The listing builds one solid part. Answer for the finished solid, in the listing's coordinates (mm). Coordinates: 2 decimals unless noted, no trailing zeros. Loops run counter-clockwise (first coordinate to the right, second up) from the corner with the lowest first, then second, coordinate; pieces in that order, holes last. Notation, with made-up numbers: (1.25, -14) - (35.25, -14) arc R35 ccw to (35.25, 23) - close; hole circle Ø4 at (-21.5, 84.5). An arc over 180 degrees is marked (long way). Write each question's results on one line, items separated by ' | '. Start each with the question number.
(1) Consider line 1 (Z direction, x = 31.5, y = 1.15); line 2 (Y direction, x = -5.5, z = 97). Determine where each line is inside the solid, lowest interval first. Write a range as from..to.
(2) Find section B-B on y = 0.8. Determine the outline of the cut face in (x, z).
(3) Find section A-A on x = 57. Determine the outline of the cut face in (y, z).
(4) Given pin 1 Ø1.5 at (x, y) = (-27, 1) entering from -Z; pin 2 Ø0.6 at (x, y) = (-23.5, 1) entering from +Z; pin 3 Ø3 at (x, z) = (-31.5, -99.5) entering from -Y, each flat-ended and moving along its own axis, determine where each tip first touches the part or whether it passes through.
from build123d import *

# Parameters (mm, degrees)
SKETCH2_W               = 140
SKETCH2_H               = 420
BOSS_EXTRUDE1_DEPTH     = 4
BOSS_EXTRUDE2_DEPTH     = 25
SKETCH4_W               = 10.25
SKETCH4_H               = 80.25
CUT_EXTRUDE1_DEPTH      = 25.4
SKETCH7_W               = 130
SKETCH7_H               = 10
CUT_EXTRUDE2_DEPTH      = 2.45
SKETCH9_W               = 140
SKETCH9_H               = 115
SKETCH9_W_2             = 10.25
SKETCH9_H_2             = 80.25
CUT_EXTRUDE3_DEPTH      = 1
CUT_EXTRUDE3_DEPTH_BACK = 30
SKETCH10_W              = 140
SKETCH10_H              = 10
BOSS_EXTRUDE3_DEPTH     = 2


with BuildPart() as part:
    # Sketch2 → Boss-Extrude1 (new body)
    with BuildSketch(Plane(origin=(0, 0, 0), x_dir=(1, 0, 0), z_dir=(0, 1, 0))):
        Rectangle(SKETCH2_W, SKETCH2_H)
    extrude(amount=BOSS_EXTRUDE1_DEPTH)

    # Sketch3 → Boss-Extrude2 (add)
    with BuildSketch(Plane(origin=(0, 4, 0), x_dir=(1, 0, 0), z_dir=(0, 1, 0))):
        with BuildLine():
            Line((-37.5, -165), (-37.5, -145))
            Line((-37.5, -145), (-43.5, -145))
            Line((-43.5, -145), (-43.5, -165))
            ThreePointArc((-43.5, -165), (0, -208.5), (43.5, -165))
            Line((43.5, -165), (43.5, -145))
            Line((43.5, -145), (37.5, -145))
            Line((37.5, -145), (37.5, -165))
            ThreePointArc((37.5, -165), (0, -202.5), (-37.5, -165))
        make_face()
    extrude(amount=BOSS_EXTRUDE2_DEPTH)

    # Sketch4 → Cut-Extrude1 (cut)
    with BuildSketch(Plane(origin=(0, 4, 0), x_dir=(1, 0, 0), z_dir=(0, 1, 0))):
        with Locations((-59.875, 139.875)):
            Rectangle(SKETCH4_W, SKETCH4_H)
        with Locations((59.875, 139.875)):
            Rectangle(SKETCH4_W, SKETCH4_H)
    extrude(amount=-CUT_EXTRUDE1_DEPTH, mode=Mode.SUBTRACT)

    # Sketch7 → Cut-Extrude2 (cut)
    with BuildSketch(Plane(origin=(0, 4, 0), x_dir=(1, 0, 0), z_dir=(0, 1, 0))):
        with Locations((0, 200)):
            Rectangle(SKETCH7_W, SKETCH7_H)
    extrude(amount=-CUT_EXTRUDE2_DEPTH, mode=Mode.SUBTRACT)

    # Sketch9 → Cut-Extrude3 (cut, two sides)
    with BuildSketch(Plane.XZ) as cut_extrude3_sk:
        with Locations((0, 152.5)):
            Rectangle(SKETCH9_W, SKETCH9_H)
        with Locations((0, -152.5)):
            Rectangle(SKETCH9_W, SKETCH9_H)
        with Locations((-59.875, -139.875)):
            Rectangle(SKETCH9_W_2, SKETCH9_H_2, mode=Mode.SUBTRACT)
        with Locations((59.875, -139.875)):
            Rectangle(SKETCH9_W_2, SKETCH9_H_2, mode=Mode.SUBTRACT)
    extrude(amount=CUT_EXTRUDE3_DEPTH, mode=Mode.SUBTRACT)
    extrude(cut_extrude3_sk.sketch, amount=-CUT_EXTRUDE3_DEPTH_BACK, mode=Mode.SUBTRACT)

    # Sketch10 → Boss-Extrude3 (add)
    with BuildSketch(Plane(origin=(0, 4, 0), x_dir=(1, 0, 0), z_dir=(0, 1, 0))):
        with Locations((0, 100)):
            Rectangle(SKETCH10_W, SKETCH10_H)
        with Locations((0, -100)):
            Rectangle(SKETCH10_W, SKETCH10_H)
    extrude(amount=-BOSS_EXTRUDE3_DEPTH)


solid = part.part
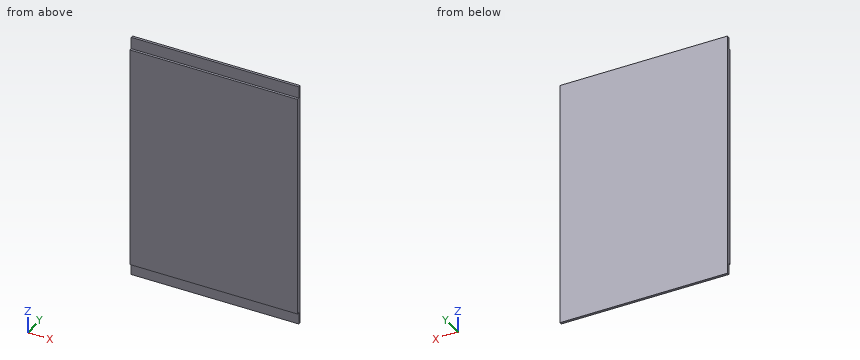
Values:
1) line 1: z = -95..95 | line 2: y = 2..4
2) outline: (-70, -95) - (70, -95) - (70, 95) - (-70, 95) - close
3) outline: (0, -95) - (2, -95) - (2, -105) - (4, -105) - (4, 105) - (2, 105) - (2, 95) - (0, 95) - close
4) pin 1: stops at z = -95 | pin 2: stops at z = 95 | pin 3: stops at y = 2
